Autodesk Inventor part; units mm, degrees
ref_plane "YZ Plane" through (0, 0, 0) normal (1, 0, 0) x (0, 1, 0)
ref_plane "XZ Plane" through (0, 0, 0) normal (0, 1, 0) x (-1, 0, 0)
ref_plane "XY Plane" through (0, 0, 0) normal (0, 0, 1) x (1, 0, 0)
sketch "Sketch1" plane through (0, 0, 0) normal (0, 0, 1) x (1, 0, 0)
  circle A0 centre (0, 0) radius 38.1
  circle A1 centre (0, 0) radius 50.8
  line L0 (-127, 25.4) -> (-127, -25.4)
  line L1 (-127, 25.4) -> (-10.3741, 49.7294)
  line L2 (-127, -25.4) -> (-10.3741, -49.7294)
  dimension "d5" = 76.2
  dimension "d6" = 101.6
  dimension "d7" = 50.8
  dimension "d8" = 127
  dimension "d9" = 25.4
extrude "Extrusion1" add sketch "Sketch1" along normal mid plane 19.05
extrude "Extrusion2" add sketch "Sketch1" along normal mid plane 38.1 contours A1
sketch "Sketch3" plane through (-127, -25.4, 9.525) normal (-1, 0, 0) x (0, 0, 1)
  line L0 (0, 50.8) -> (31.75, 50.8)
  line L1 (0, 0) -> (31.75, 0)
  arc A0 (31.75, 0) -> (31.75, 50.8) centre (31.75, 25.4) ccw
  line L2 (-19.05, 0) -> (-19.05, 50.8)
  circle A1 centre (31.75, 25.4) radius 12.7
  line L3 (0, 50.8) -> (0, 0)
  line L4 (0, 50.8) -> (-19.05, 50.8)
  point P0 (-9.525, 25.4)
  dimension "d14" = 25.4
  dimension "d15" = 50.8
  dimension "d16" = 25.4
extrude "Extrusion3" add sketch "Sketch3" against normal blind 25.4
properties part number "HW 7 Part 4" material "Aluminum 6061"
Part model, mm, in its own coordinate system. A direction names the side the tool comes from. Give positions to 0.01 mm unless a question says otherwise; leave off trailing zeros. Loops run counter-clockwise (first coordinate to the right, second up) from the corner with the lowest first, then second, coordinate; pieces in that order, holes last. Notation, with made-up numbers: M 29,31.5 L 40,31.5 A11 ccw 40,39.5 Z; hole C 41.5,2 d3. An arc over 180 degrees is marked long. Return JSON: item names as keys, results as strings.
1) Saw through at B-B, the plane y = 0. List the corners of the cut face in (x, z) (3 decimals), then the cut area to 3 significant figures.
Calculated:
{"outline": "M -127,-9.525 L -50.8,-9.525 L -50.8,-19.05 L -38.1,-19.05 L -38.1,19.05 L -50.8,19.05 L -50.8,9.525 L -101.6,9.525 L -101.6,28.575 L -127,28.575 Z; M -127,53.975 L -101.6,53.975 L -101.6,66.675 L -127,66.675 Z; M 38.1,-19.05 L 50.8,-19.05 L 50.8,19.05 L 38.1,19.05 Z", "area": "3,230 mm2"}
2) 3-axis set-ups, long thin cutter, end or side, ignore diameter. For faces 5 (the face through (-69.503, -37.394, -0.133)), 6 (the face through (-127, 0, 20)), 7 (the face through (-114, -25.4, 25)), 8 (the face through (-114, 25.4, 25)), 9 (the face through (-101.6, 0, 25)): which of +Z, -Z, +X, -X, +Y, -Y reach the whole face in a straight line?
Calculated:
{"face 5": "+Z, -Z, -X, -Y", "face 6": "+Z, -Z, -X, +Y, -Y", "face 7": "+Z, -X, -Y", "face 8": "+Z, -X, +Y", "face 9": "+Z, +Y, -Y"}
3) Pull direction Y, two halves, no side cores. Call faces 1 (the face through (-69.503, 37.394, -0.133)), 2 (the face through (-114.48, -0.56, 66.67)), 3 (the face through (7, 38, 19.05)), 4 (the face through (-114.478, 0.558, 28.587)): released by +Y, released by -Y, zero draft, split by the parting line, or undercut.
Calculated:
{"face 1": "released by +Y", "face 2": "split by the parting line", "face 3": "zero draft", "face 4": "undercut"}
4) Flat gauge pins, fed straight in: pin 1 Ø1.5 at (x, z) = (9.5, 4) entering from -Y; pin 2 Ø1 at (x, z) = (-14.5, 13) entering from -Y; pin 3 Ø20.5 at (x, z) = (-111.5, 27) entering from +Y; pin 4 Ø12 at (x, y) = (-13, 31.5) entering from -Z. Where does each tip first touch, or does it go through?
Calculated:
{"pin 1": "stops at y = -50.04", "pin 2": "stops at y = -48.83", "pin 3": "stops at y = 25.4", "pin 4": "stops at z = -19.05"}
5) Saw through at D-D, the plane z = 2.5. List the corners of the cut face in (x, y), then the cut area to 3 significant figures.
Calculated:
{"outline": "M -127,-25.4 L -10.37,-49.73 A50.8 ccw long -10.37,49.73 L -127,25.4 Z; hole C 0,0 d76.2", "area": "9,300 mm2"}
6) Saw through at C-C, the plane x = 0. List the corners of the cut face in (y, z), then the cut area to 3 significant figures.
Calculated:
{"outline": "M -50.8,-19.05 L -38.1,-19.05 L -38.1,19.05 L -50.8,19.05 Z; M 38.1,-19.05 L 50.8,-19.05 L 50.8,19.05 L 38.1,19.05 Z", "area": "968 mm2"}
7) Saw through at A-A, the plane z = 13. List the corners of the cut face in (x, y), then the cut area to 3 significant figures.
Calculated:
{"outline": "M -127,-25.4 L -101.6,-25.4 L -101.6,25.4 L -127,25.4 Z; C 0,0 d101.6; hole C 0,0 d76.2", "area": "4,840 mm2"}
8) Drill centre lines: line 1 (Y direction, x = 0, z = -5); line 2 (Z direction, x = 33, y = -23); line 3 (X direction, y = 3, z = -15). Where is each one in solid material? Low to high.
Calculated:
{"line 1": "y = -50.8 to -38.1, 38.1 to 50.8", "line 2": "z = -19.05 to 19.05", "line 3": "x = -50.71 to -37.98, 37.98 to 50.71"}
